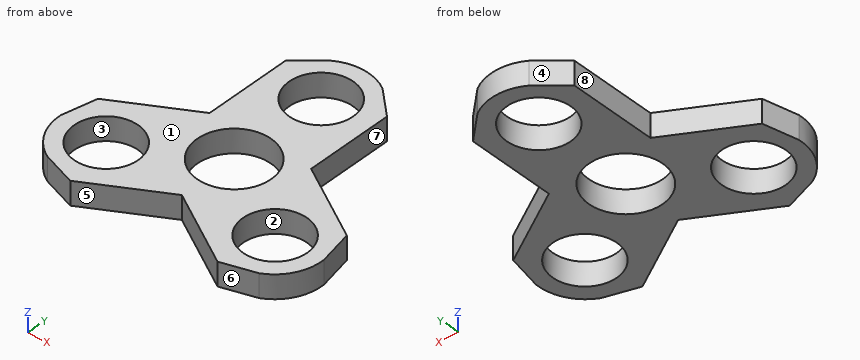
```python
from build123d import *

# Parameters (mm, degrees)
SKETCH2_R             = 10.975
SKETCH2_R_2           = 9.5
BOSS_EXTRUDE1_DEPTH   = 7
BODY_MOVE_COPY2_ANGLE = 90


with BuildPart() as part:
    # Sketch2 → Boss-Extrude1 (new body)
    with BuildSketch(Plane(origin=(0, 0, 0), x_dir=(1, 0, 0), z_dir=(0, 1, 0))):
        with BuildLine():
            Line((15.1, 8.717989065), (15.1, 34))
            Line((15.1, 34), (7.646696155, 40.860405367))
            ThreePointArc((7.646696155, 40.860405367), (0.033272999, 43.046889297), (-7.548090014, 40.751707603))
            Line((-7.548090014, 40.751707603), (-15.1, 34))
            Line((-15.1, 34), (-15.1, 8.717989065))
            Line((-15.1, 8.717989065), (-36.994863729, -3.923016403))
            Line((-36.994863729, -3.923016403), (-39.209497135, -13.807969558))
            ThreePointArc((-39.209497135, -13.807969558), (-37.296336185, -21.494629386), (-31.517969025, -26.912691504))
            Line((-31.517969025, -26.912691504), (-21.894863729, -30.076983597))
            Line((-21.894863729, -30.076983597), (0, -17.43597813))
            Line((0, -17.43597813), (21.894863729, -30.076983597))
            Line((21.894863729, -30.076983597), (31.562800979, -27.052435809))
            ThreePointArc((31.562800979, -27.052435809), (37.263063186, -21.552259911), (39.066059039, -13.8390161))
            Line((39.066059039, -13.8390161), (36.994863729, -3.923016403))
            Line((36.994863729, -3.923016403), (15.1, 8.717989065))
        make_face()
        Circle(SKETCH2_R, mode=Mode.SUBTRACT)
        with Locations((0, 29)):
            Circle(SKETCH2_R_2, mode=Mode.SUBTRACT)
        with Locations((25.11473671, -14.5)):
            Circle(SKETCH2_R_2, mode=Mode.SUBTRACT)
        with Locations((-25.11473671, -14.5)):
            Circle(SKETCH2_R_2, mode=Mode.SUBTRACT)
    extrude(amount=BOSS_EXTRUDE1_DEPTH)


with BuildPart() as part_1:
    # Body-Move/Copy2: moved
    add(part.part.rotate(Axis((0, 3.5, -6.485131953), (1, 0, 0)), BODY_MOVE_COPY2_ANGLE))


solid = part_1.part
```
Geometry: final body of the model. Coordinates: model frame, mm. Face numbers are marked on the shaded views. A direction names the side the tool comes from. Coordinates: 2 decimals unless noted, no trailing zeros. Order: outer loops, then holes, each group sorted by start corner. A loop starts at its lowest first (then second) coordinate and runs counter-clockwise, first axis right, second up. Notation, with made-up numbers: (41.25, -34) -> (71.25, -34) arc R22 ccw to (71.25, -9) -> close; hole circle Ø2 at (48, 54.5). An arc over 180 degrees is marked (long way). Answer in a Markdown table with one row per item.
Item 1: Access query for the marked faces 5, 6, 7 and 8. Directions: +Z, -Z, +X, -X, +Y, -Y. A direction counts if a zero-diameter tool reaches every point of the face in a straight line with its end or side. Return the directions, or none.
Return value:
| item | result |
|---|---|
| face 5 | +Z, -Z, -Y |
| face 6 | +Z, -Z, +X, -Y |
| face 7 | +Z, -Z, +X, +Y |
| face 8 | +Z, -Z, -X, +Y |
Item 2: Section B-B on x = 4.5. Output: boundary loops of the cut face in (y, z).
Return value:
| item | result |
|---|---|
| outline | (-23.02, -9.99) -> (-13, -9.99) -> (-13, -2.99) -> (-23.02, -2.99) -> close; (7.02, -9.99) -> (17.65, -9.99) -> (17.65, -2.99) -> (7.02, -2.99) -> close; (34.38, -9.99) -> (39.36, -9.99) -> (39.36, -2.99) -> (34.38, -2.99) -> close |
Item 3: Draft query along Y for the marked faces 1, 2, 3 and 4. Return one class per face: released by +Y, released by -Y, zero draft, split by the parting line, or undercut.
Return value:
| item | result |
|---|---|
| face 1 | zero draft |
| face 2 | undercut |
| face 3 | undercut |
| face 4 | released by +Y |
Item 4: Contact query for flat-ended pins moving along their axis: P1, Ø11.5, axis at x = -25.11, y = -17.49, coming from the +Z side; P2, Ø3, axis at x = 17, z = -7.5, coming from the +Y side; P3, Ø2, axis at y = -5.5, z = -8.5, coming from the +X side; P4, Ø8, axis at x = -3.5, y = 18.5, coming from the -Z side. Output: stop coordinate, or through.
Return value:
| item | result |
|---|---|
| P1 | passes through |
| P2 | stops at y = 5.5 |
| P3 | stops at x = 36.29 |
| P4 | stops at z = -9.99 |
Item 5: Section D-D on x = 28.5. Output: boundary loops of the cut face in (y, z), plus the area to 3 significant figures.
Return value:
| item | result |
|---|---|
| outline | (-31, -9.99) -> (-26.36, -9.99) -> (-26.36, -2.99) -> (-31, -2.99) -> close; (-8.61, -9.99) -> (-2, -9.99) -> (-2, -2.99) -> (-8.61, -2.99) -> close |
| area | 78.7 mm² |
Item 6: Ray query, L1, parallel to Y at x = 0, z = -5; L2, parallel to Y at x = -6.5, z = -7.25; L3, parallel to X at y = -22.5, z = -8.75. Return the intervals inside material, ascending.
Return value:
| item | result |
|---|---|
| L1 | y = -20.42 to -13.96, 7.99 to 16.51, 35.51 to 40.06 |
| L2 | y = -24.17 to -11.83, 5.86 to 19.09, 32.94 to 38.39 |
| L3 | x = -38.26 to -33.18, -17.05 to -3.6, 3.6 to 17.05, 33.18 to 38.21 |
Item 7: Section A-A on x = -24.5. Output: boundary loops of the cut face in (y, z).
Return value:
| item | result |
|---|---|
| outline | (-32.21, -9.99) -> (-26.97, -9.99) -> (-26.97, -2.99) -> (-32.21, -2.99) -> close; (-8.01, -9.99) -> (0.31, -9.99) -> (0.31, -2.99) -> (-8.01, -2.99) -> close |
Item 8: Section C-C on z = -7. State how many separate pieces and enclosed holes the cut face has, plus the area to 3 significant figures.
Return value:
| item | result |
|---|---|
| separate pieces | 1 |
| enclosed holes | 4 |
| area | 1,990 mm² |
